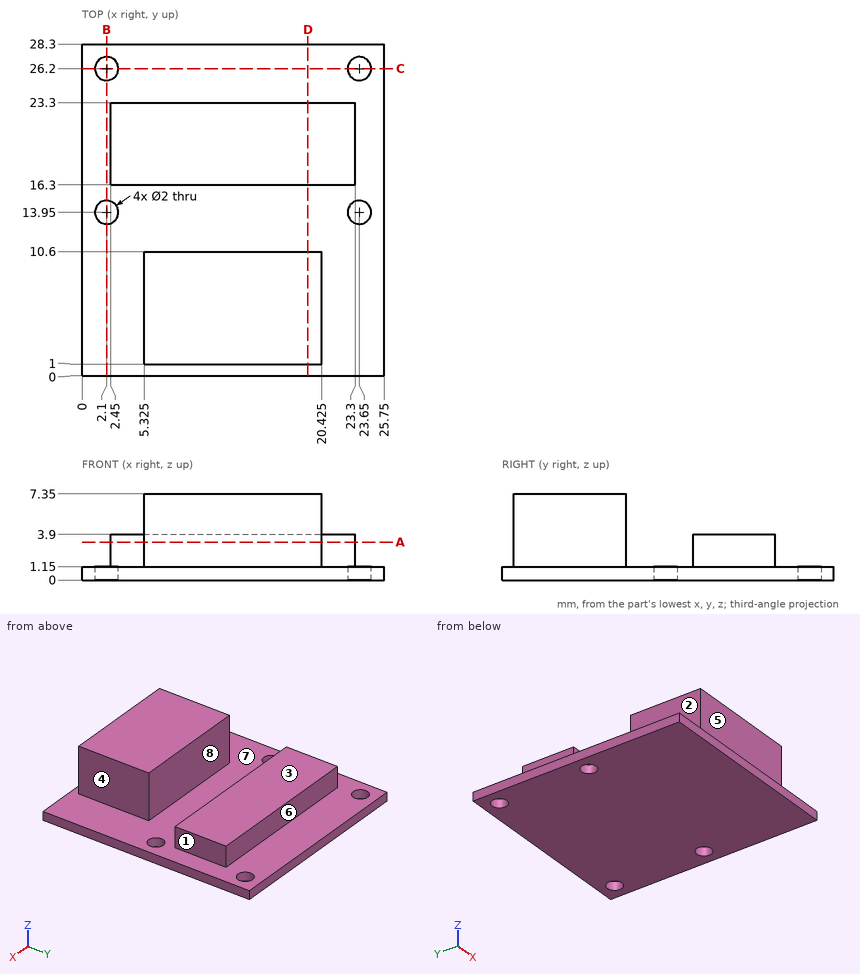
Study the drawing (mm; zero at the part's minimum x, y, z) and answer. A direction names the side the tool comes from. Coordinates: 2 decimals unless noted, no trailing zeros. Write each loop counter-clockwise with the first axis right and the second up, starting at its lowest first coordinate (ties: lowest second). Pieces come first, ordered by that corner, then holes. Notation, with made-up numbers: (-20.75, 84.5) - (-3.75, 84.5) arc R21 ccw to (-3.75, 107.5) - close; hole circle Ø5 at (39.25, 44). An arc over 180 degrees is marked (long way). Return JSON: item names as keys, results as strings. Group by question number.
1. Determine the mould class of the marked faces 5, 6, 7 and 8 for opening direction Y: released by +Y, released by -Y, zero draft, split by the parting line, or undercut.
2. Given pin 1 (1.4 mm diameter, centred on y = 21, z = 3, fed in from +X); pin 2 (2 mm diameter, centred on x = 12, y = 21.5, fed in from +Z); pin 3 (3 mm diameter, centred on y = 5, z = 5.5, fed in from +X) (3 decimals); pin 4 (1.6 mm diameter, centred on x = 23.65, y = 13.95, fed in from -Z), each flat-ended and moving along its own axis, determine where each tip first touches the part or whether it passes through.
3. A cutting plane is placed at D-D, the plane x = 19.25. Determine the outline of the cut face in (y, z), plus the area to 3 significant figures.
4. Straight lines are drawn through the part: L1, parallel to Y at x = 23.65, z = 0.4; L2, parallel to Z at x = 2.25, y = 2.5; L3, parallel to X at y = 5.5, z = 3.25 (3 decimals). For each, find the intervals that lie inside material, in ascending order.
5. A cutting plane is placed at C-C, the plane y = 26.2. Determine the outline of the cut face in (x, z).
6. A cutting plane is placed at A-A, the plane z = 3.25. Determine the outline of the cut face in (x, y) (3 decimals).
7. A cutting plane is placed at B-B, the plane x = 2.1. Determine the outline of the cut face in (y, z), plus the area to 3 significant figures.
8. Which of the six approach directions +Z, -Z, +X, -X, +Y, -Y give full straight-line access (tool end or side, diameter ignored) to the marked faces 1, 2, 3 and 4?
Ans:
{
 "1": {"face 5": "released by -Y", "face 6": "released by +Y", "face 7": "undercut", "face 8": "undercut"},
 "2": {"pin 1": "x = 23.3", "pin 2": "z = 3.9", "pin 3": "x = 20.425", "pin 4": "through"},
 "3": {"outline": "(0, 0) - (28.3, 0) - (28.3, 1.15) - (23.3, 1.15) - (23.3, 3.9) - (16.3, 3.9) - (16.3, 1.15) - (10.6, 1.15) - (10.6, 7.35) - (1, 7.35) - (1, 1.15) - (0, 1.15) - close", "area": "111 mm²"},
 "4": {"L1": "0 to 12.95, 14.95 to 25.2, 27.2 to 28.3", "L2": "0 to 1.15", "L3": "5.325 to 20.425"},
 "5": {"outline": "(0, 0) - (1.1, 0) - (1.1, 1.15) - (0, 1.15) - close; (3.1, 0) - (22.65, 0) - (22.65, 1.15) - (3.1, 1.15) - close; (24.65, 0) - (25.75, 0) - (25.75, 1.15) - (24.65, 1.15) - close"},
 "6": {"outline": "(2.45, 16.3) - (23.3, 16.3) - (23.3, 23.3) - (2.45, 23.3) - close; (5.325, 1) - (20.425, 1) - (20.425, 10.6) - (5.325, 10.6) - close"},
 "7": {"outline": "(0, 0) - (12.95, 0) - (12.95, 1.15) - (0, 1.15) - close; (14.95, 0) - (25.2, 0) - (25.2, 1.15) - (14.95, 1.15) - close; (27.2, 0) - (28.3, 0) - (28.3, 1.15) - (27.2, 1.15) - close", "area": "27.9 mm²"},
 "8": {"face 1": "+Z, +X, +Y, -Y", "face 2": "+Z, -X, -Y", "face 3": "+Z, +X, -X, +Y", "face 4": "+Z, +X, -Y"}
}
